Check sheet for the drawn part. Datum: minimum x, y, z corner. Units: mm. A direction names the side the tool comes from. Round coordinates to 2 decimals unless told otherwise and drop trailing zeros. Write each loop counter-clockwise with the first axis right and the second up, starting at its lowest first coordinate (ties: lowest second). Pieces come first, ordered by that corner, then holes. Notation, with made-up numbers: (-5.75, 76.5) -> (37.25, 76.5) arc R18 ccw to (37.25, 99.5) -> close; hole circle Ø3 at (77.5, -39.75). An arc over 180 degrees is marked (long way). One line per item, written item: value.
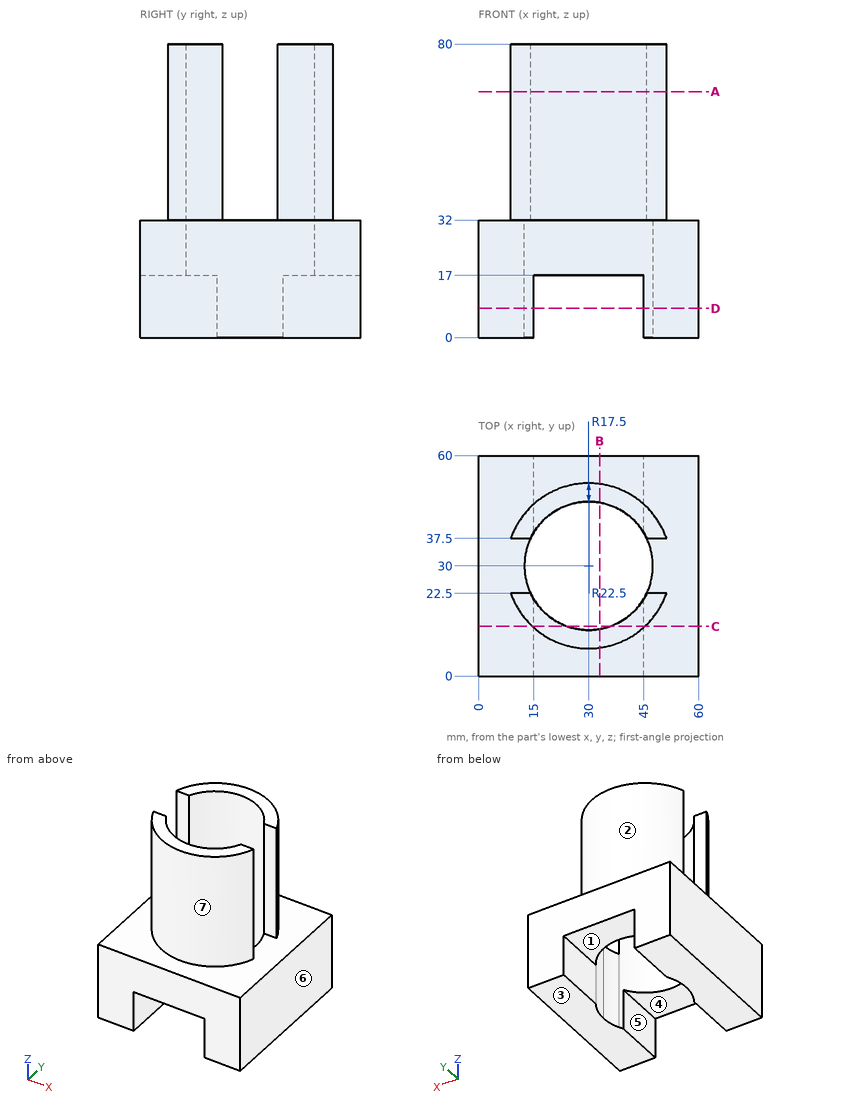
Item 1: Thickness scan on line 1 (X direction, y = 39, z = 20); line 2 (Y direction, x = 37.5, z = 44); line 3 (Y direction, x = 46, z = 74). Record the ranges inside material, lowest first.
Answer:
line 1: x = 0 to 14.99, 45.01 to 60
line 2: y = 8.79 to 14.19, 45.81 to 51.21
line 3: y = 14.18 to 22.5, 37.5 to 45.82
Item 2: Depth check by flat-ended pin: P1, Ø10.5, axis at x = 27.5, y = 48.5, coming from the -Z side; P2, Ø5, axis at x = 51, z = 40.5, coming from the +Y side; P3, Ø1.6, axis at x = 12, z = 54, coming from the -Y side. Enter the tip coordinate at first touch or a pass-through.
Answer:
P1: stops at z = 17
P2: stops at y = 42.81
P3: stops at y = 15.49
Item 3: Sectioned sample at A-A on z = 67. Enter the section's corners in (x, y), and give its area (3 significant figures).
Answer:
outline: (8.79, 22.5) arc R22.5 ccw to (51.21, 22.5) -> (45.81, 22.5) arc R17.5 cw to (14.19, 22.5) -> close; (8.79, 37.5) -> (14.19, 37.5) arc R17.5 cw to (45.81, 37.5) -> (51.21, 37.5) arc R22.5 ccw to start
area: 474 mm^2
Item 4: Sectioned sample at B-B on x = 33. Enter the section's corners in (y, z), and give its area (3 significant figures).
Answer:
outline: (0, 17) -> (12.76, 17) -> (12.76, 80) -> (7.7, 80) -> (7.7, 32) -> (0, 32) -> close; (47.24, 17) -> (60, 17) -> (60, 32) -> (52.3, 32) -> (52.3, 80) -> (47.24, 80) -> close
area: 868 mm^2
Item 5: Mould release check, pull along X, two halves, no side actions. Record for the marked faces 1, 2, 3 and 4: pulls with the +X half, pulls with the -X half, needs draft (parallel to the pull), parting line crosses it, or undercut.
Answer:
face 1: undercut
face 2: parting line crosses it
face 3: needs draft
face 4: undercut
Item 6: Sectioned sample at D-D on z = 8. Enter the section's corners in (x, y), and give its area (3 significant figures).
Answer:
outline: (0, 0) -> (15, 0) -> (15, 20.99) arc R17.5 cw to (14.19, 22.5) arc R17.5 cw to (14.19, 37.5) arc R17.5 cw to (15, 39.01) -> (15, 60) -> (0, 60) -> close; (45, 0) -> (60, 0) -> (60, 60) -> (45, 60) -> (45, 39.01) arc R17.5 cw to (45.81, 37.5) arc R17.5 cw to (47.5, 30) arc R17.5 cw to (45.81, 22.5) arc R17.5 cw to (45, 20.99) -> close
area: 1,740 mm^2
Item 7: Tool access check on the marked faces 5, 6 and 7. Record the directions out of +Z, -Z, +X, -X, +Y, -Y that give a thin tool (end or side, any length) a straight path to the whole face; none if there is none.
Answer:
face 5: -Z, +Y, -Y
face 6: +Z, -Z, +X, +Y, -Y
face 7: +Z, -Y
Item 8: Sectioned sample at C-C on y = 13.5. Enter the section's corners in (x, z), and give its area (3 significant figures).
Answer:
outline: (0, 0) -> (15, 0) -> (15, 17) -> (24.17, 17) -> (24.17, 80) -> (14.7, 80) -> (14.7, 32) -> (0, 32) -> close; (35.83, 17) -> (45, 17) -> (45, 0) -> (60, 0) -> (60, 32) -> (45.3, 32) -> (45.3, 80) -> (35.83, 80) -> close
area: 2,140 mm^2
